The listing builds one solid part. Answer for the finished solid, in the listing's coordinates (mm). Round coordinates to 2 decimals unless told otherwise and drop trailing zeros. Order: outer loops, then holes, each group sorted by start corner. A loop starts at its lowest first (then second) coordinate and runs counter-clockwise, first axis right, second up. Notation, with made-up numbers: (-10, 38.25) - (33, 38.25) arc R25 cw to (33, 71.25) - close; hole circle Ø2 at (-5, 85). An arc over 180 degrees is marked (long way). Write item = value, one per line.
from build123d import *

# Parameters (mm, degrees)
BOSS_EXTRUDE1_DEPTH = 2.5
FILLET2_R           = 0.3
FILLET3_R           = 0.3


with BuildPart() as part:
    # Sketch1 → Boss-Extrude1 (new body)
    with BuildSketch(Plane(origin=(0, 0, 0), x_dir=(1, 0, 0), z_dir=(0, 1, 0))):
        with BuildLine():
            ThreePointArc((3.9, 0), (-2.987573328, -2.506871678), (0.677227893, 3.840750237))
            ThreePointArc((0.677227893, 3.840750237), (1.89360662, 4.692467791), (1.041889066, 5.908846518))
            ThreePointArc((1.041889066, 5.908846518), (-4.596266659, -3.856725658), (6, 0))
            ThreePointArc((6, 0), (4.95, 1.05), (3.9, 0))
        make_face()
    extrude(amount=BOSS_EXTRUDE1_DEPTH)

    # Fillet2
    fillet2_edges = [part.edges().sort_by_distance(p)[0] for p in [
        (1.89360662, 2.5, -4.692467791),
        (-4.596266659, 2.5, 3.856725658),
        (4.95, 2.5, -1.05),
        (-2.987573328, 2.5, 2.506871678),
    ]]
    fillet(fillet2_edges, radius=FILLET2_R)

    # Fillet3
    fillet3_edges = [part.edges().sort_by_distance(p)[0] for p in [
        (-4.596266659, 0, 3.856725658),
        (1.89360662, 0, -4.692467791),
        (-2.987573328, 0, 2.506871678),
        (4.95, 0, -1.05),
    ]]
    fillet(fillet3_edges, radius=FILLET3_R)


solid = part.part
Q1. Section A-A on y = 1.8 is taken. Determine the outline of the cut face in (x, z), then the cut area to 3 significant figures.
Model answer:
outline = (0.68, -3.84) arc R3.9 cw (long way) to (3.9, 0) arc R1.05 ccw to (6, 0) arc R6 ccw (long way) to (1.04, -5.91) arc R1.05 ccw to start
area = 54.3 mm^2
Q2. Find the intervals of material crossed by line 1 (X direction, y = 1.7, z = 0); line 2 (X direction, y = 2.1, z = 2.75), in increasing order. Write a range as from..to.
Model answer:
line_1 = -6..-3.9, 3.9..6
line_2 = -5.33..-2.77, 2.77..5.33
Q3. Determine the mould class of faces 1 (the face through (-4, 2.5, 2)), 2 (the face through (1.89, 1.24, -4.67)), 3 (the face through (4.97, 1.24, -1.05)), 4 (the face through (-2.9, 1.24, 2.61)) for opening direction Z: released by +Z, released by -Z, zero draft, split by the parting line, or undercut.
Model answer:
face_1 = zero draft
face_2 = undercut
face_3 = released by -Z
face_4 = undercut
